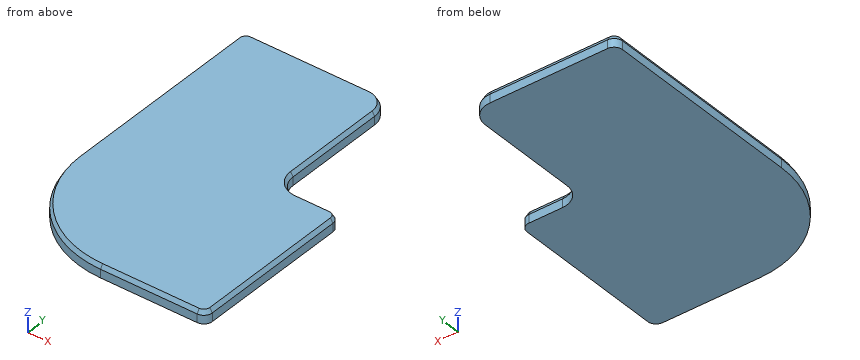
```python
from build123d import *

# Parameters (mm, degrees)
F1_DEPTH = 3
F2_SIZE2 = 0.57735
F2_SIZE  = 1


with BuildPart() as f1:
    # F0 (on Top) → F1 (new body)
    with BuildSketch(Plane.XY):
        with BuildLine():
            Line((0, 32.6), (0, 0))
            Line((0, 0), (0, -15.4))
            ThreePointArc((0, -15.4), (7.32233, -33.07767), (25, -40.4))
            Line((25, -40.4), (48, -40.4))
            ThreePointArc((48, -40.4), (49.414214, -39.814214), (50, -38.4))
            Line((50, -38.4), (50, -2))
            ThreePointArc((50, -2), (49.414214, -0.585786), (48, 0))
            Line((48, 0), (40, 0))
            ThreePointArc((40, 0), (36.464466, 1.464466), (35, 5))
            Line((35, 5), (35, 29.6))
            ThreePointArc((35, 29.6), (33.535534, 33.135534), (30, 34.6))
            Line((30, 34.6), (2, 34.6))
            ThreePointArc((2, 34.6), (0.585786, 34.014214), (0, 32.6))
        make_face()
    extrude(amount=F1_DEPTH)

    # F2
    f2_edges = [f1.edges().sort_by_distance(p)[0] for p in [
        (0, 8.6, 3),
    ]]
    chamfer(f2_edges, length=F2_SIZE, length2=F2_SIZE2)


solid = f1.part
```
Model file for the job. Use its own axes, mm. Coordinates: 2 decimals unless noted, no trailing zeros. Order: outer loops, then holes, each group sorted by start corner. A loop starts at its lowest first (then second) coordinate and runs counter-clockwise, first axis right, second up. Notation, with made-up numbers: (78.5, 7) -> (108.5, 7) arc R8 cw to (108.5, 14) -> close; hole circle Ø6 at (46, -20.75). An arc over 180 degrees is marked (long way). Return JSON: item names as keys, results as strings.
Item 1: Slice it at B-B (y = 17). Write the cut outline in (x, z).
Model answer:
{"outline": "(0, 0) -> (35, 0) -> (35, 2) -> (34.42, 3) -> (0.58, 3) -> (0, 2) -> close"}
Item 2: Pin check, flat tips, straight feed: P1, Ø8, axis at x = 41, y = 22, coming from the -Z side; P2, Ø1.5, axis at y = 10.5, z = 2.5, coming from the -X side; P3, Ø0.6, axis at x = 43, z = 1, coming from the +Y side; P4, Ø0.6, axis at y = 22.5, z = 1.5, coming from the +X side. Stop position of each tip, or through.
Model answer:
{"P1": "passes through", "P2": "stops at x = 0", "P3": "stops at y = 0", "P4": "stops at x = 35"}
Item 3: Slice it at A-A (z = 1.05). Write the cut outline in (x, y).
Model answer:
{"outline": "(0, -15.4) arc R25 ccw to (25, -40.4) -> (48, -40.4) arc R2 ccw to (50, -38.4) -> (50, -2) arc R2 ccw to (48, 0) -> (40, 0) arc R5 cw to (35, 5) -> (35, 29.6) arc R5 ccw to (30, 34.6) -> (2, 34.6) arc R2 ccw to (0, 32.6) -> close"}
Item 4: Wall check: line 1 along X through (y, z) = (20, 1.5); line 2 along Y through (x, z) = (43.5, 0.45); line 3 along Y through (x, z) = (10.5, 1.95). Give the ranges that are in metal, low to high. Write a range as from..to.
Model answer:
{"line 1": "x = 0..35", "line 2": "y = -40.4..0", "line 3": "y = -35.77..34.6"}
Item 5: Slice it at C-C (x = 46.5). Write the cut outline in (y, z), then the cut area to 3 significant figures.
Model answer:
{"outline": "(-40.4, 0) -> (0, 0) -> (0, 2) -> (-0.58, 3) -> (-39.82, 3) -> (-40.4, 2) -> close", "area": "121 mm²"}
